The listing builds one solid part. Answer for the finished solid, in the listing's coordinates (mm). Give positions to 0.01 mm unless a question says otherwise; leave off trailing zeros. Loops run counter-clockwise (first coordinate to the right, second up) from the corner with the lowest first, then second, coordinate; pieces in that order, holes last. Notation, with made-up numbers: M 43.5,76 L 66.5,76 A20 ccw 66.5,103 Z; hole C 17,-1.5 d6. An arc over 180 degrees is marked long. Use one line per item in the form item = value. Start each with the question number.
1. The mould has two halves that part along Y. Classify faces 1 (the face through (3.29, 3.38, 37.86)), 2 (the face through (8, 50.8, 19)), 3 (the face through (16.352, 50.281, 19.306)): released by +Y, released by -Y, zero draft, split by the parting line, or undercut.
2. The part is cut by section A-A (z = 30.5). Write down the section's boundary in (x, y) (1 decimal).
3. Straight lines are drawn through the part: line 1 (Y direction, x = 5, z = 10); line 2 (Y direction, x = 5.25, z = 5.5); line 3 (X direction, y = 44.5, z = 15). For each, find the intervals that lie inside material, in ascending order. Write a range as from..to.
4. Each of these flat-tipped pins is pushed along its axis until it touches: pin 1 Ø1.5 at (x, y) = (7.5, 39) entering from -Z; pin 2 Ø4 at (y, z) = (15.5, 34) entering from +X; pin 3 Ø4.5 at (x, y) = (4.76, 7.94) entering from -Z; pin 4 Ø5 at (x, z) = (3.5, 7) entering from -Y. Where does it stop, or does it pass through?
from build123d import *

# Parameters (mm, degrees)
BOSS_EXTRUDE1_DEPTH = 38.1
SKETCH2_R           = 1.905
CUT_EXTRUDE1_DEPTH  = 66.935388863
CHAMFER1_SIZE       = 6.35
FILLET1_R           = 0.79375
CHAMFER2_SIZE       = 0.79375


with BuildPart() as part:
    # Sketch1 → Boss-Extrude1 (new body)
    with BuildSketch(Plane.XY):
        with BuildLine():
            Line((0, 0), (17.754591081, 0))
            ThreePointArc((17.754591081, 0), (5.55625, 25.4), (17.754591081, 50.8))
            Line((17.754591081, 50.8), (0, 50.8))
            Line((0, 50.8), (0, 0))
        make_face()
    extrude(amount=BOSS_EXTRUDE1_DEPTH)

    # Sketch2 → Cut-Extrude1 (cut, through all)
    with BuildSketch(Plane.XY.offset(38.1)):
        with Locations((4.7625, 46.0375)):
            Circle(SKETCH2_R)
        with Locations((4.7625, 7.9375)):
            Circle(SKETCH2_R)
    extrude(amount=-CUT_EXTRUDE1_DEPTH, mode=Mode.SUBTRACT)

    # Chamfer1
    chamfer1_edges = [part.edges().sort_by_distance(p)[0] for p in [
        (0, 0, 19.05),
    ]]
    chamfer(chamfer1_edges, length=CHAMFER1_SIZE)

    # Fillet1
    fillet1_edges = [part.edges().sort_by_distance(p)[0] for p in [
        (5.55625, 25.4, 38.1),
        (8.877295541, 50.8, 38.1),
        (12.052295541, 0, 0),
        (12.052295541, 0, 38.1),
        (6.35, 0, 19.05),
        (3.175, 3.175, 0),
        (0, 6.35, 19.05),
        (3.175, 3.175, 38.1),
        (0, 28.575, 38.1),
        (8.877295541, 50.8, 0),
        (5.55625, 25.4, 0),
        (0, 28.575, 0),
        (0, 50.8, 19.05),
        (17.754591081, 50.8, 19.05),
        (17.754591081, 0, 19.05),
    ]]
    fillet(fillet1_edges, radius=FILLET1_R)

    # Chamfer2
    chamfer2_edges = [part.edges().sort_by_distance(p)[0] for p in [
        (2.8575, 46.0375, 0),
        (2.8575, 46.0375, 38.1),
        (2.8575, 7.9375, 0),
        (2.8575, 7.9375, 38.1),
    ]]
    chamfer(chamfer2_edges, length=CHAMFER2_SIZE)


solid = part.part
Derived:
q1.face_1 = released by -Y
q1.face_2 = released by +Y
q1.face_3 = undercut
q2.outline = M 0,6.7 A0.8 ccw 0.2,6.1 L 6.1,0.2 A0.8 ccw 6.7,0 L 15.6,0 A0.8 ccw 16.1,1.4 A32.5 cw 16.1,49.4 A0.8 ccw 15.6,50.8 L 0.8,50.8 A0.8 ccw 0,50 Z; hole C 4.8,7.9 d3.8; hole C 4.8,46 d3.8
q3.line_1 = 1.35..6.05, 9.83..44.15, 47.93..50.8
q3.line_2 = 1.1..6.1, 9.78..44.2, 47.88..50.8
q3.line_3 = 0..3.64, 5.89..11.75
q4.pin_1 = 0
q4.pin_2 = 7.81
q4.pin_3 = 0.45
q4.pin_4 = 0.35
